Can you work these out from the model? Positions are in its coordinate system, mm. Give positions to 0.01 mm unless a question says otherwise; leave off trailing zeros. Loops run counter-clockwise (first coordinate to the right, second up) from the corner with the lowest first, then second, coordinate; pieces in that order, holes last. Notation, with made-up numbers: (-30, 32.25) - (-26, 32.25) arc R13 ccw to (-26, 47.25) - close; hole circle Ø5 at (-21, 7). An arc over 180 degrees is marked (long way). Answer in a Markdown table with one row per item.
from build123d import *

# Parameters (mm, degrees)
F0_R        = 11.2
F1_DEPTH    = 7
F2_T1_DEPTH = 111.6025403784
F2_T3_DEPTH = 111.6025403784
F2_T5_DEPTH = 111.6025403784
F3_T1_DEPTH = 106.6025403784
F3_T3_DEPTH = 106.6025403784
F3_T5_DEPTH = 106.6025403784


# Not quite as in the source:
# - a fillet or chamfer that OpenCascade refuses, or shapes differently, is made with other operations: its cross-section is extruded or revolved along the edge and cut away or added


with BuildPart() as f1:
    # F0 (on Top) → F1 (new body)
    with BuildSketch(Plane.XY):
        Polygon((43.3012701892, -25), (0, 50), (-43.3012701892, -25), align=None)
        with Locations((-20.4962927973, -11.8335401639)):
            Circle(F0_R, mode=Mode.SUBTRACT)
        with Locations((20.4962927973, -11.8335401639)):
            Circle(F0_R, mode=Mode.SUBTRACT)
        Circle(F0_R, mode=Mode.SUBTRACT)
        with Locations((0, 23.6670803279)):
            Circle(F0_R, mode=Mode.SUBTRACT)
    extrude(amount=F1_DEPTH)

    # F2: fillet of radius 5 on 3 edges, made by hand

    # F2_s2 → F2_t1 (cut)
    with BuildSketch(Plane(origin=(27.9006350946, 48.3253175473, 0), x_dir=(0, 0, 1), z_dir=(-0.5, -0.8660254038, 0))):
        with BuildLine():
            ThreePointArc((2, 25), (5.5355339059, 23.5355339059), (7, 20))
            Line((7, 20), (7, 25))
            Line((7, 25), (2, 25))
        make_face()
    extrude(amount=F2_T1_DEPTH, mode=Mode.SUBTRACT)

    # F2_s4 → F2_t3 (cut)
    with BuildSketch(Plane.YZ.offset(-55.8012701892)):
        with BuildLine():
            ThreePointArc((-25, 2), (-23.5355339059, 5.5355339059), (-20, 7))
            Line((-20, 7), (-25, 7))
            Line((-25, 7), (-25, 2))
        make_face()
    extrude(amount=F2_T3_DEPTH, mode=Mode.SUBTRACT)

    # F2_s6 → F2_t5 (cut)
    with BuildSketch(Plane(origin=(27.9006350946, -48.3253175473, 0), x_dir=(0, 0, 1), z_dir=(-0.5, 0.8660254038, 0))):
        with BuildLine():
            ThreePointArc((2, 25), (5.5355339059, 23.5355339059), (7, 20))
            Line((7, 20), (7, 25))
            Line((7, 25), (2, 25))
        make_face()
    extrude(amount=F2_T5_DEPTH, mode=Mode.SUBTRACT)

    # F3: fillet of radius 5 on 3 edges, made by hand

    # F3_s2 → F3_t1 (cut)
    with BuildSketch(Plane(origin=(26.6506350946, -46.1602540378, 0), x_dir=(0, 0, 1), z_dir=(-0.5, 0.8660254038, 0))):
        with BuildLine():
            ThreePointArc((2, 25), (0.527864045, 23.2360679775), (0, 21))
            Line((0, 21), (0, 25))
            Line((0, 25), (2, 25))
        make_face()
    extrude(amount=F3_T1_DEPTH, mode=Mode.SUBTRACT)

    # F3_s4 → F3_t3 (cut)
    with BuildSketch(Plane.YZ.offset(-53.3012701892)):
        with BuildLine():
            ThreePointArc((-21, 0), (-23.2360679775, 0.527864045), (-25, 2))
            Line((-25, 2), (-25, 0))
            Line((-25, 0), (-21, 0))
        make_face()
    extrude(amount=F3_T3_DEPTH, mode=Mode.SUBTRACT)

    # F3_s6 → F3_t5 (cut)
    with BuildSketch(Plane(origin=(26.6506350946, 46.1602540378, 0), x_dir=(0, 0, 1), z_dir=(-0.5, -0.8660254038, 0))):
        with BuildLine():
            ThreePointArc((0, 21), (0.527864045, 23.2360679775), (2, 25))
            Line((2, 25), (0, 25))
            Line((0, 25), (0, 21))
        make_face()
    extrude(amount=F3_T5_DEPTH, mode=Mode.SUBTRACT)


solid = f1.part
Q1. Imagine slicing it at A-A, the plane z = 5.75. Write out the boundary of the cut face in (x, y).
Checked values:
| item | result |
|---|---|
| outline | (-40.37, -23.31) - (40.37, -23.31) - (0, 46.61) - close; hole circle Ø22.4 at (-20.5, -11.83); hole circle Ø22.4 at (0, 0); hole circle Ø22.4 at (0, 23.67); hole circle Ø22.4 at (20.5, -11.83) |
Q2. If we mould it in two halves opening along X, with no side actions, what happens to faces 1 (the face through (-11, 4, 7)), 2 (the face through (-11.19, 0.49, 3.45)), 3 (the face through (20.84, 11.33, 0.8))? For each: released by +X, released by -X, zero draft, split by the parting line, or undercut.
Checked values:
| item | result |
|---|---|
| face 1 | zero draft |
| face 2 | undercut |
| face 3 | released by +X |
Q3. If I drill on line 1 (Y direction, x = 2, z = 1.75); line 2 (Y direction, x = -5, z = 2.75); line 3 (X direction, y = -18.5, z = 5.75), over which ranges is the centre line in solid material (lowest first)? Write a range as [from, to].
Checked values:
| item | result |
|---|---|
| line 1 | y = [-24.8, -11.02], [11.02, 12.65], [34.69, 46.14] |
| line 2 | y = [-24.94, -10.02], [10.02, 13.65], [33.69, 41.23] |
| line 3 | x = [-37.59, -29.5], [-11.5, 11.5], [29.5, 37.59] |
Q4. Imagine slicing it at B-B, the plane x = 1.5. Count the separate pieces of the cut face and the enclosed holes in it, and give its area (3 significant figures).
Checked values:
| item | result |
|---|---|
| separate pieces | 3 |
| enclosed holes | 0 |
| area | 173 mm² |
Q5. For pin 1 (3 mm diameter, centred on y = 20, z = 2.5, fed in from -X); pin 2 (1 mm diameter, centred on y = 15, z = 1, fed in from -X); pin 3 (13.5 mm diameter, centred on x = -20.5, y = -11.83, fed in from -Z); pin 4 (4 mm diameter, centred on x = 23.5, y = 6, fed in from +Z), each with a flat end and sliding along its axis, tell me the tip position at first contact or that it passes through.
Checked values:
| item | result |
|---|---|
| pin 1 | stops at x = -18.17 |
| pin 2 | stops at x = -19.78 |
| pin 3 | passes through |
| pin 4 | stops at z = 6.81 |
